Design review of the part built by this model. Coordinates are the model's own, in mm. Face numbers are marked on the shaded views. A direction names the side the tool comes from. Give positions to 0.01 mm unless a question says otherwise; leave off trailing zeros. Loops run counter-clockwise (first coordinate to the right, second up) from the corner with the lowest first, then second, coordinate; pieces in that order, holes last. Notation, with made-up numbers: (-8.5, 57) -> (42.5, 57) arc R19 cw to (42.5, 73) -> close; hole circle Ø7 at (58, -25). An arc over 180 degrees is marked (long way). Answer as CSV lines item,"result".
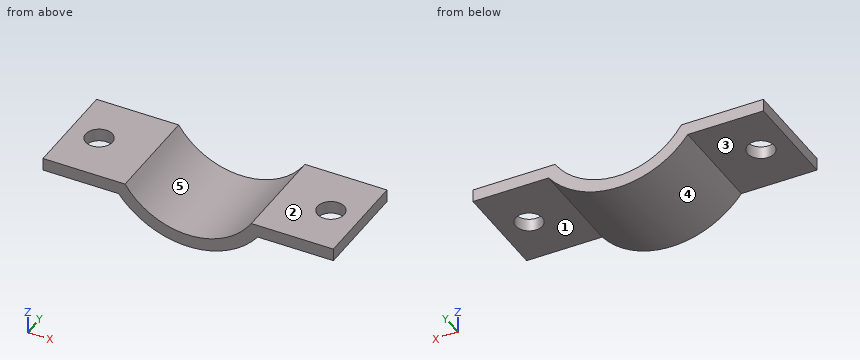
from build123d import *

# Parameters (mm, degrees)
SKETCH1_R           = 19.05
BOSS_EXTRUDE1_DEPTH = 25.4
SKETCH2_R           = 3.3782
CUT_EXTRUDE1_DEPTH  = 36.8775
SKETCH3_W           = 85.242997218
SKETCH3_H           = 34.152222548
CUT_EXTRUDE2_DEPTH  = 26.4


with BuildPart() as part:
    # Sketch1 → Boss-Extrude1 (new body)
    with BuildSketch(Plane(origin=(0, 0, 0), x_dir=(1, 0, 0), z_dir=(0, 1, 0))):
        with BuildLine():
            Line((36.587384889, 13.6525), (17.537384889, 13.6525))
            ThreePointArc((17.537384889, 13.6525), (0, 22.225), (-17.537384889, 13.6525))
            Line((-17.537384889, 13.6525), (-36.587384889, 13.6525))
            Line((-36.587384889, 13.6525), (-36.587384889, 4.1275))
            Line((-36.587384889, 4.1275), (-21.838369187, 4.1275))
            ThreePointArc((-21.838369187, 4.1275), (0, -22.225), (21.838369187, 4.1275))
            Line((21.838369187, 4.1275), (36.587384889, 4.1275))
            Line((36.587384889, 4.1275), (36.587384889, 13.6525))
        make_face()
        Circle(SKETCH1_R, mode=Mode.SUBTRACT)
    extrude(amount=BOSS_EXTRUDE1_DEPTH)

    # Sketch2 → Cut-Extrude1 (cut, through all)
    with BuildSketch(Plane(origin=(0, 0, -13.6525), x_dir=(-1, 0, 0), z_dir=(0, 0, -1))):
        with Locations((29.21, 12.7)):
            Circle(SKETCH2_R)
        with Locations((-29.21, 12.7)):
            Circle(SKETCH2_R)
    extrude(amount=-CUT_EXTRUDE1_DEPTH, mode=Mode.SUBTRACT)

    # Sketch3 → Cut-Extrude2 (cut, through all)
    with BuildSketch(Plane(origin=(0, 25.4, 0), x_dir=(1, 0, 0), z_dir=(0, 1, 0))):
        with Locations((-0.146640147, -6.598611274)):
            Rectangle(SKETCH3_W, SKETCH3_H)
    extrude(amount=-CUT_EXTRUDE2_DEPTH, mode=Mode.SUBTRACT)


solid = part.part
Q1. Clearance check with flat-ended pins moving along their axes: pin 1 Ø1 at (x, y) = (-12.5, 6) entering from -Z; pin 2 Ø5 at (x, y) = (-11, 19) entering from +Z; pin 3 Ø8 at (x, y) = (3.5, 16.5) entering from -Z (3 decimals). State where each tip first meets the part, or that it passes through.
Filled sheet:
pin 1,"stops at z = -18.71"
pin 2,"stops at z = -13.44"
pin 3,"stops at z = -22.225"
Q2. The part is to be moulded in two halves that separate along X. For the marked faces 3, 4 and 5, say which applies: pulls with the +X half, pulls with the -X half, needs draft (parallel to the pull), parting line crosses it, or undercut.
Filled sheet:
face 3,"needs draft"
face 4,"parting line crosses it"
face 5,"undercut"
Q3. We need section B-B, the plane y = 12.7. State how many separate pieces and enclosed holes the cut face has, and give its area (3 significant figures).
Filled sheet:
separate pieces,"3"
enclosed holes,"0"
area,"207 mm^2"
Q4. To check wall thickness, follow probe 1 along Y at (x, z) = (-29.21, -11.15); probe 2 along Z at (x, y) = (29.5, 2.5); probe 3 along X at (y, z) = (14.5, -14.75). State the ranges of each line that lie inside material, in increasing order. Write a range as from..to.
Filled sheet:
probe 1,"y = 0..9.32, 16.08..25.4"
probe 2,"z = -13.65..-10.48"
probe 3,"x = -16.62..-12.06, 12.06..16.62"
Q5. We need section C-C, the plane z = -17.25. State the section outline as (x, y) points, and give its area (3 significant figures).
Filled sheet:
outline,"(-14.01, 0) -> (-8.08, 0) -> (-8.08, 25.4) -> (-14.01, 25.4) -> close; (8.08, 0) -> (14.01, 0) -> (14.01, 25.4) -> (8.08, 25.4) -> close"
area,"301 mm^2"
Q6. For the marked faces 1 and 2, list the 3-axis set-ups (+Z, -Z, +X, -X, +Y, -Y) from which the entire face can be reached by the end or side of a thin tool; tool diameter is ignored.
Filled sheet:
face 1,"-Z, +X, +Y, -Y"
face 2,"+Z, +X, -X, +Y, -Y"
Q7. We need section A-A, the plane x = -29.21. State the section outline as (y, z) points.
Filled sheet:
outline,"(0, -13.65) -> (9.32, -13.65) -> (9.32, -10.48) -> (0, -10.48) -> close; (16.08, -13.65) -> (25.4, -13.65) -> (25.4, -10.48) -> (16.08, -10.48) -> close"
